Model file for the job. Use its own axes, mm. A direction names the side the tool comes from. Round coordinates to 2 decimals unless told otherwise and drop trailing zeros. Order: outer loops, then holes, each group sorted by start corner. A loop starts at its lowest first (then second) coordinate and runs counter-clockwise, first axis right, second up. Notation, with made-up numbers: (6, 80.25) - (55, 80.25) arc R23 cw to (55, 109.25) - close; hole circle Ø11 at (34, -13.75). An arc over 180 degrees is marked (long way). Put each result on its own line as item: value. Start each with the question number.
Item 1: Pin check, flat tips, straight feed: pin 1 Ø1.5 at (y, z) = (0, 3.5) entering from -X; pin 2 Ø2.5 at (x, y) = (-7.93, 43.58) entering from -Z; pin 3 Ø8 at (y, z) = (-17.5, 2.5) entering from -X. Stop position of each tip, or through.
Item 2: Saw through at A-A on x = -50.5. List the corners of the cut face in (y, z), plus the area to 3 significant figures.
Item 3: Saw through at D-D on x = -73. List the corners of the cut face in (y, z), plus the area to 3 significant figures.
Item 4: Probe probe 1 along Y at (x, z) = (-47, 17.75); probe 2 along X at (y, z) = (44, 7.25); probe 3 along Z at (x, y) = (-24, 12.5). List the from-to ranges inside material, lowest first.
Item 5: Which spindle directions (+Z, -Z, +X, -X, +Y, -Y) get a long thin tool onto all of the face, cutting with end or side? Do faces 4 (the face through (-110.82, 25.9, 9.48)), 5 (the face through (-32, 24, 6.35)), 6 (the face through (-14.315, 60.884, 15.831)). Say none if no direction does.
Item 6: Saw through at C-C on z = 10.5. List the corners of the cut face in (x, y) (3 decimals), plus the area to 3 significant figures.
Item 7: Saw through at B-B on y = 19. List the corners of the cut face in (x, z), plus the area to 3 significant figures.
Item 8: Mould opens along X. For faces 1 (the face through (34.822, 47.663, 3.131)), 2 (the face through (-30, -21, 12.7)), 3 (the face through (-8.211, 45.732, 9.569)) say: pulls with the +X half, pulls with the -X half, needs draft (parallel to the pull), parting line crosses it, or undercut.
```python
from build123d import *

# Parameters (mm, degrees)
SKETCH1_R           = 82.296
SKETCH1_R_2         = 57.15
SKETCH1_R_3         = 4.191
BOSS_EXTRUDE1_DEPTH = 6.35
SKETCH2_R           = 67.211414491
SKETCH2_R_2         = 9.525
BOSS_EXTRUDE2_DEPTH = 6.35
SKETCH3_R           = 9.525
SKETCH3_R_2         = 17.4625
BOSS_EXTRUDE3_DEPTH = 6.35
SKETCH4_R           = 2.15265
SKETCH4_R_2         = 2.169226356
CUT_EXTRUDE1_DEPTH  = 13.97


with BuildPart() as part:
    # Sketch1 → Boss-Extrude1 (new body)
    with BuildSketch(Plane.XY):
        with Locations((-43.673560496, 22.943742375)):
            Circle(SKETCH1_R)
        with Locations((-43.673560496, 22.943742375)):
            Circle(SKETCH1_R_2, mode=Mode.SUBTRACT)
        with Locations((-98.06108088, 73.910708897)):
            Circle(SKETCH1_R_3, mode=Mode.SUBTRACT)
        with Locations((7.293406026, 77.331262758)):
            Circle(SKETCH1_R_3, mode=Mode.SUBTRACT)
        with Locations((10.713959888, -28.023224148)):
            Circle(SKETCH1_R_3, mode=Mode.SUBTRACT)
        with Locations((-94.640527019, -31.443778009)):
            Circle(SKETCH1_R_3, mode=Mode.SUBTRACT)
    extrude(amount=BOSS_EXTRUDE1_DEPTH)

    # Sketch2 → Boss-Extrude2 (add)
    with BuildSketch(Plane.XY.offset(6.35)):
        with Locations((-43.673560496, 22.943742375)):
            Circle(SKETCH2_R)
        with Locations((-43.673560496, 22.943742375)):
            Circle(SKETCH2_R_2, mode=Mode.SUBTRACT)
    extrude(amount=BOSS_EXTRUDE2_DEPTH)

    # Sketch3 → Boss-Extrude3 (add)
    with BuildSketch(Plane.XY.offset(12.7)):
        with BuildLine():
            Line((-3.962770655, 42.915113639), (-24.961079117, 79.362585794))
            ThreePointArc((-24.961079117, 79.362585794), (-43.673560496, 90.155156865), (-62.386041875, 79.362585794))
            Line((-62.386041875, 79.362585794), (-82.148620619, 45.202948303))
            ThreePointArc((-82.148620619, 45.202948303), (-44.973677355, -21.487240016), (-3.962770655, 42.915113639))
        make_face()
        with Locations((-43.673560496, 22.943742375)):
            Circle(SKETCH3_R, mode=Mode.SUBTRACT)
        with Locations((-43.673560496, 68.536742375)):
            Circle(SKETCH3_R_2, mode=Mode.SUBTRACT)
    extrude(amount=BOSS_EXTRUDE3_DEPTH)

    # Sketch4 → Cut-Extrude1 (cut)
    with BuildSketch(Plane.XY.offset(12.7)):
        with Locations((-79.418759037, 43.581242375)):
            Circle(SKETCH4_R)
        with Locations((-7.928361955, 43.581242375)):
            Circle(SKETCH4_R_2)
        with Locations((-43.673560496, -18.331257625)):
            Circle(SKETCH4_R)
    extrude(amount=-CUT_EXTRUDE1_DEPTH, mode=Mode.SUBTRACT)


solid = part.part
```
Results found:
1. pin 1: stops at x = -122.92
1. pin 2: stops at z = 12.7
1. pin 3: stops at x = -117.46
2. outline: (-59.07, 0) - (-33.8, 0) - (-33.8, 6.35) - (16.3, 6.35) - (16.3, 19.05) - (-20.98, 19.05) - (-20.98, 12.7) - (-43.92, 12.7) - (-43.92, 6.35) - (-59.07, 6.35) - close; (29.59, 6.35) - (79.68, 6.35) - (79.68, 0) - (104.96, 0) - (104.96, 6.35) - (89.81, 6.35) - (89.81, 12.7) - (89.05, 12.7) - (89.05, 19.05) - (84.61, 19.05) - (84.61, 12.7) - (52.46, 12.7) - (52.46, 19.05) - (29.59, 19.05) - close
2. area: 1,500 mm²
3. outline: (-53.95, 0) - (-26.11, 0) - (-26.11, 6.35) - (72, 6.35) - (72, 0) - (99.84, 0) - (99.84, 6.35) - (83.42, 6.35) - (83.42, 12.7) - (61.02, 12.7) - (61.02, 19.05) - (-10.46, 19.05) - (-10.46, 12.7) - (-37.53, 12.7) - (-37.53, 6.35) - (-53.95, 6.35) - close
3. area: 1,580 mm²
4. probe 1: y = -21.38 to 14.02, 31.87 to 51.39, 85.68 to 89.9
4. probe 2: x = -107.5 to -81.53, -77.31 to -10.06, -5.8 to 20.15
4. probe 3: z = 6.35 to 19.05
5. face 4: +Z
5. face 5: -Z
5. face 6: +Z, +X, +Y
6. outline: circle Ø134.423 at (-43.674, 22.944); hole circle Ø4.305 at (-79.419, 43.581); hole circle Ø19.05 at (-43.674, 22.944); hole circle Ø4.305 at (-43.674, -18.331); hole circle Ø4.338 at (-7.928, 43.581)
6. area: 13,900 mm²
7. outline: (-125.88, 0) - (-100.69, 0) - (-100.69, 6.35) - (-52.34, 6.35) - (-52.34, 19.05) - (-87.95, 19.05) - (-87.95, 12.7) - (-110.77, 12.7) - (-110.77, 6.35) - (-125.88, 6.35) - close; (-35, 6.35) - (13.34, 6.35) - (13.34, 0) - (38.53, 0) - (38.53, 6.35) - (23.42, 6.35) - (23.42, 12.7) - (0.6, 12.7) - (0.6, 19.05) - (-35, 19.05) - close
7. area: 1,510 mm²
8. face 1: parting line crosses it
8. face 2: needs draft
8. face 3: undercut
